```python
from build123d import *

# Parameters (mm, degrees)
F1_DEPTH  = 60
F3_DEPTH  = 5
F5_DEPTH  = 5.001
F7_DEPTH  = 5.001
F9_DEPTH  = 60.001
F11_REACH = 66.0565127546
F12_R     = 9.999


# Not quite as in the source:
# - a fillet or chamfer is up to 0.001 mm smaller than in the source, because OpenCascade refuses the exact size


with BuildPart() as f1:
    # F0 (on Front) → F1 (new body)
    with BuildSketch(Plane.XZ):
        with BuildLine():
            Line((-30, 0), (30, 0))
            ThreePointArc((30, 0), (0, 30), (-30, 0))
        make_face()
    extrude(amount=F1_DEPTH)

    # F2 (on face) → F3 (join)
    with BuildSketch(Plane(origin=(0, 0, 0), x_dir=(1, 0, 0), z_dir=(0, 0, -1))):
        with BuildLine():
            ThreePointArc((-40, 20), (-50, 10), (-40, 0))
            Line((-40, 0), (40, 0))
            ThreePointArc((40, 0), (50, 10), (40, 20))
            Line((40, 20), (-40, 20))
        make_face()
    extrude(amount=-F3_DEPTH)

    # F4 (on face) → F5 (cut, through all)
    with BuildSketch(Plane.XY.offset(5)):
        with BuildLine():
            Line((-45, -10), (-40, -10))
            Line((-40, -10), (-40, -5))
            ThreePointArc((-40, -5), (-43.5355339059, -6.4644660941), (-45, -10))
        make_face()
        with BuildLine():
            Line((-40, -5), (-40, -10))
            Line((-40, -10), (-35, -10))
            ThreePointArc((-35, -10), (-36.4644660941, -6.4644660941), (-40, -5))
        make_face()
        with BuildLine():
            Line((-40, -10), (-40, -15))
            ThreePointArc((-40, -15), (-36.4644660941, -13.5355339059), (-35, -10))
            Line((-35, -10), (-40, -10))
        make_face()
        with BuildLine():
            ThreePointArc((-45, -10), (-43.5355339059, -13.5355339059), (-40, -15))
            Line((-40, -15), (-40, -10))
            Line((-40, -10), (-45, -10))
        make_face()
    extrude(amount=-F5_DEPTH, mode=Mode.SUBTRACT)

    # F6 (on face) → F7 (cut, through all)
    with BuildSketch(Plane.XY.offset(5)):
        with BuildLine():
            ThreePointArc((40, -5), (36.4644660941, -6.4644660941), (35, -10))
            Line((35, -10), (40, -10))
            Line((40, -10), (40, -5))
        make_face()
        with BuildLine():
            Line((40, -5), (40, -10))
            Line((40, -10), (45, -10))
            ThreePointArc((45, -10), (43.5355339059, -6.4644660941), (40, -5))
        make_face()
        with BuildLine():
            Line((45, -10), (40, -10))
            Line((40, -10), (40, -15))
            ThreePointArc((40, -15), (43.5355339059, -13.5355339059), (45, -10))
        make_face()
        with BuildLine():
            Line((40, -10), (35, -10))
            ThreePointArc((35, -10), (36.4644660941, -13.5355339059), (40, -15))
            Line((40, -15), (40, -10))
        make_face()
    extrude(amount=-F7_DEPTH, mode=Mode.SUBTRACT)

    # F8 (on face) → F9 (cut, through all)
    with BuildSketch(Plane.XZ.offset(60)):
        with BuildLine():
            Line((-20, 0), (20, 0))
            ThreePointArc((20, 0), (0, 20), (-20, 0))
        make_face()
    extrude(amount=-F9_DEPTH, mode=Mode.SUBTRACT)

    f11_end = f1.faces().sort_by_distance((0, -30, 30))[0]
    # F10 (on Top) → F11 (cut, up to a face of the model that its end follows)
    with BuildSketch(Plane.XY):
        Polygon((-10, -60), (0, -60), (10, -60), (10, -30), (-10, -30), align=None)
    f11_long = extrude(amount=F11_REACH, mode=Mode.PRIVATE)
    add(split(f11_long, bisect_by=f11_end, keep=Keep.BOTTOM, mode=Mode.PRIVATE), mode=Mode.SUBTRACT)

    # F12 (radius 10 in the source; OpenCascade refuses exactly that, so slightly less here)
    f12_edges = [f1.edges().sort_by_distance(p)[0] for p in [
        (-10, -30, 22.80239),
        (10, -30, 22.80239),
    ]]
    fillet(f12_edges, radius=F12_R)


solid = f1.part
```
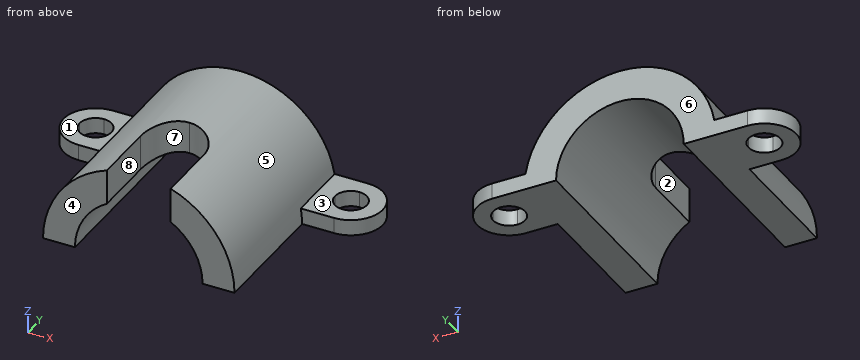
Input: part model. Units: mm. Frame: model coordinates. Face numbers are marked on the shaded views. A direction names the side the tool comes from. Coordinates: 2 decimals unless noted, no trailing zeros. Loops run counter-clockwise (first coordinate to the right, second up) from the corner with the lowest first, then second, coordinate; pieces in that order, holes last. Notation, with made-up numbers: M -3,62 L 5,62 A18 cw 5,86 Z; hole C 39.25,-33 d9. An arc over 180 degrees is marked long. Answer in a Markdown table with one row per item.
1. Reachability of the marked faces 1, 2, 3 and 4 from +Z, -Z, +X, -X, +Y, -Y: full face, straight path, thin tool, end or side. Return the list, or none.
Response:
| item | result |
|---|---|
| face 1 | +Z, -X, +Y, -Y |
| face 2 | +Z, -Z, -Y |
| face 3 | +Z, +X, +Y, -Y |
| face 4 | +Z, -Z, +X, -X, -Y |
2. Section C-C, the plane z = 10.5. Output: boundary loops of the cut face in (x, y).
Response:
| item | result |
|---|---|
| outline | M -28.1,-60 L -17.02,-60 L -17.02,0 L -28.1,0 Z; M 17.02,-60 L 28.1,-60 L 28.1,0 L 17.02,0 Z |
3. Section D-D, the plane y = -25.5. Output: boundary loops of the cut face in (x, z).
Response:
| item | result |
|---|---|
| outline | M -30,0 L -20,0 A20 cw 20,0 L 30,0 A30 ccw Z |
4. Draft query along X for the marked faces 5, 6, 7 and 8. Return one class per face: pulls with the +X half, pulls with the -X half, needs draft (parallel to the pull), parting line crosses it, or undercut.
Response:
| item | result |
|---|---|
| face 5 | parting line crosses it |
| face 6 | needs draft |
| face 7 | undercut |
| face 8 | undercut |
5. Material intervals for line 1 (X direction, y = -52.5, z = 15); line 2 (X direction, y = -17, z = 4); line 3 (Z direction, x = -27.5, y = -8.5), sorted ascending.
Response:
| item | result |
|---|---|
| line 1 | x = -25.98 to -13.23, 13.23 to 25.98 |
| line 2 | x = -47.14 to -19.6, 19.6 to 47.14 |
| line 3 | z = 0 to 11.99 |
6. First-contact query: pin 1 (16 mm diameter, centred on x = -43.5, y = -8, fed in from +Z); pin 2 (2 mm diameter, centred on y = -16.5, z = 10.5, fed in from +X); pin 3 (8 mm diameter, centred on x = -21, y = -12.5, fed in from +Z). Flat tips, straight axial feed; report the tip coordinate or a pass-through.
Response:
| item | result |
|---|---|
| pin 1 | stops at z = 5 |
| pin 2 | stops at x = 28.46 |
| pin 3 | stops at z = 24.72 |
7. Section A-A, the plane y = -48. Output: boundary loops of the cut face in (x, z), then the cut area to 3 significant figures.
Response:
| item | result |
|---|---|
| outline | M -30,0 L -20,0 A20 cw -10,17.32 L -10,28.28 A30 ccw Z; M 10,17.32 A20 cw 20,0 L 30,0 A30 ccw 10,28.28 Z |
| area | 579 mm2 |
